The listing builds one solid part. Answer for the finished solid, in the listing's coordinates (mm). Round coordinates to 2 decimals unless told otherwise and drop trailing zeros. Write each loop counter-clockwise with the first axis right and the second up, starting at its lowest first coordinate (ties: lowest second). Pieces come first, ordered by that corner, then holes. Notation, with made-up numbers: M 87,54.25 L 134,54.25 A25 ccw 134,70.25 Z; hole C 4,-32 d7. An arc over 180 degrees is marked long. Put each result on its own line as item: value. Start each with the question number.
```python
from build123d import *

# Parameters (mm, degrees)
CROQUIS1_R              = 385.3
SALIENTE_EXTRUIR1_DEPTH = 543.2
CROQUIS3_R              = 50
CROQUIS2_R              = 385.3
CROQUIS4_R              = 50
SALIENTE_EXTRUIR2_DEPTH = 100


# Read off the part's stored shape, not the designer's step: Vaciado1
with BuildPart() as part:
    # Croquis1 → Saliente-Extruir1 (new body)
    with BuildSketch(Plane(origin=(0, 0, 0), x_dir=(1, 0, 0), z_dir=(0, 1, 0))):
        with Locations(Location((0, 0, 0), (0, 0, 270))):
            Circle(CROQUIS1_R)
    extrude(amount=-SALIENTE_EXTRUIR1_DEPTH)

    # Croquis3 → Recubrir1 section 0
    with BuildSketch(Plane(origin=(0, -878.5, 0), x_dir=(1, 0, 0), z_dir=(0, 1, 0))):
        Circle(CROQUIS3_R)
    # Croquis2 → Recubrir1 section 1
    with BuildSketch(Plane.XZ.offset(543.2)):
        Circle(CROQUIS2_R)
    loft()

    # Croquis4 → Saliente-Extruir2 (add)
    with BuildSketch(Plane.XZ.offset(878.5)):
        with Locations(Location((0, 0, 0), (0, 0, 270))):
            Circle(CROQUIS4_R)
    extrude(amount=SALIENTE_EXTRUIR2_DEPTH)

    # Vaciado1 outline → Vaciado1 (revolve, cut)
    with BuildSketch(Plane.XY):
        Polygon((382.125, -541.884871939), (382.125, 0), (0, 0), (0, -978.5), (46.825, -978.5), (46.825, -877.184871939), align=None)
    revolve(axis=Axis((0, 0, 0), (0, 1, 0)), mode=Mode.SUBTRACT)


solid = part.part
```
Item 1: Consider line 1 along X through (y, z) = (-909.5, 0) (3 decimals); line 2 along X through (y, z) = (-428.5, 0) (3 decimals). Determine where each line is inside the solid, lowest interval first. Write a range as [from, to].
Item 2: Section C-C (y = -774.5) is taken. Give the vertices of the cut face in (x, z).
Item 3: Section B-B (y = -163.5) is taken. Give the vertices of the cut face in (x, z) (3 decimals), and give its area (3 significant figures).
Item 4: Determine the mould class of faces 1 (the cylindrical face through (364.48, -267.15, -114.78)), 2 (the flat face through (-15, -978.5, 45)), 3 (the cylindrical face through (15.02, -927.8, -47.69)) for opening direction Z: released by +Z, released by -Z, zero draft, split by the parting line, or undercut.
Item 5: Flat-ended cylindrical pins translate along their axes: pin 1 (8 mm diameter, centred on x = -155.5, z = 250, fed in from -Y); pin 2 (6 mm diameter, centred on x = 108.5, y = -335.5, fed in from -Z) (3 decimals); pin 3 (2 mm diameter, centred on y = -879, z = -30.5, fed in from +X). Find the tip coordinate at first contact, or state that the pin passes through.
Output values:
1. line 1: x = [-50, -46.825], [46.825, 50]
1. line 2: x = [-385.3, -382.125], [382.125, 385.3]
2. outline: C 0,0 d308; hole C 0,0 d299.02
3. outline: C 0,0 d770.6; hole C 0,0 d764.25
3. area: 7,650 mm^2
4. face 1: undercut
4. face 2: zero draft
4. face 3: split by the parting line
5. pin 1: stops at y = -638.08
5. pin 2: stops at z = -370.575
5. pin 3: stops at x = 40.46
